For this review, take the finished solid that the model builds, in its own axes (mm). Round coordinates to 2 decimals unless told otherwise and drop trailing zeros. Write each loop counter-clockwise with the first axis right and the second up, starting at its lowest first coordinate (ties: lowest second). Pieces come first, ordered by that corner, then holes. Notation, with made-up numbers: M -11.75,-19.5 L 18.25,-19.5 A6 ccw 18.25,-15.5 Z; hole C -27.75,24 d7. An arc over 180 degrees is marked long. One line per question, with ' | ' between items.
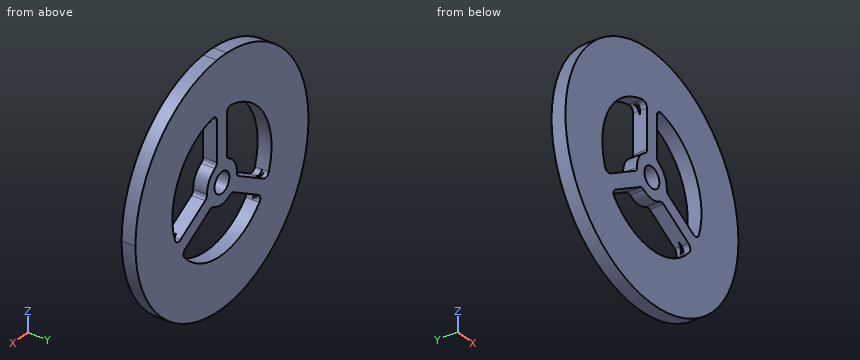
```python
from build123d import *

# Parameters (mm, degrees)
F0_R     = 1.5
F1_DEPTH = 1


with BuildPart() as f1:
    # F0 (on Front) → F1 (new body, symmetric)
    with BuildSketch(Plane.XZ):
        with BuildLine():
            ThreePointArc((-1, 17.412308), (-11.973877, -12.681275), (17.441, 0))
            ThreePointArc((17.441, 0), (12.681275, 11.973877), (1, 17.412308))
            ThreePointArc((1, 17.412308), (0, 17.441), (-1, 17.412308))
        make_face()
        with BuildLine():
            ThreePointArc((-2.373679, -2.525145), (-1.983172, -2.424438), (-1.596733, -2.539773))
            ThreePointArc((-1.596733, -2.539773), (0, -3), (1.596733, -2.539773))
            ThreePointArc((1.596733, -2.539773), (1.983172, -2.424438), (2.373679, -2.525145))
            Line((2.373679, -2.525145), (7.363259, -5.40588))
            ThreePointArc((7.363259, -5.40588), (7.729194, -5.933007), (7.555614, -6.550779))
            ThreePointArc((7.555614, -6.550779), (0, -10), (-7.555614, -6.550779))
            ThreePointArc((-7.555614, -6.550779), (-7.729194, -5.933007), (-7.363259, -5.40588))
            Line((-7.363259, -5.40588), (-2.373679, -2.525145))
        make_face(mode=Mode.SUBTRACT)
        with BuildLine():
            ThreePointArc((-9.450948, -3.267964), (-8.660254, 5), (-1.895334, 9.818743))
            ThreePointArc((-1.895334, 9.818743), (-1.273538, 9.660182), (-1, 9.079709))
            Line((-1, 9.079709), (-1, 3.318238))
            ThreePointArc((-1, 3.318238), (-1.108039, 2.929697), (-1.401141, 2.652697))
            ThreePointArc((-1.401141, 2.652697), (-2.598076, 1.5), (-2.997874, -0.112925))
            ThreePointArc((-2.997874, -0.112925), (-3.091211, -0.505258), (-3.373679, -0.793094))
            Line((-3.373679, -0.793094), (-8.363259, -3.673829))
            ThreePointArc((-8.363259, -3.673829), (-9.002732, -3.727174), (-9.450948, -3.267964))
        make_face(mode=Mode.SUBTRACT)
        Circle(F0_R, mode=Mode.SUBTRACT)
        with BuildLine():
            Line((1, 3.318238), (1, 9.079709))
            ThreePointArc((1, 9.079709), (1.273538, 9.660182), (1.895334, 9.818743))
            ThreePointArc((1.895334, 9.818743), (8.660254, 5), (9.450948, -3.267964))
            ThreePointArc((9.450948, -3.267964), (9.002732, -3.727174), (8.363259, -3.673829))
            Line((8.363259, -3.673829), (3.373679, -0.793094))
            ThreePointArc((3.373679, -0.793094), (3.091211, -0.505258), (2.997874, -0.112925))
            ThreePointArc((2.997874, -0.112925), (2.598076, 1.5), (1.401141, 2.652697))
            ThreePointArc((1.401141, 2.652697), (1.108039, 2.929697), (1, 3.318238))
        make_face(mode=Mode.SUBTRACT)
    extrude(amount=F1_DEPTH, both=True)

    # F2 (on Right) → F3 (revolve, cut)
    with BuildSketch(Plane.YZ):
        Polygon((0.4216, 9.94), (0, 10), (0, 8.5), align=None)
    revolve(axis=Axis((0, -2.204443, 0), (0, 1, 0)), mode=Mode.SUBTRACT)


solid = f1.part
```
Item 1: To check wall thickness, follow line 1 along X through (y, z) = (0.6, -3.5); line 2 along Z through (x, y) = (-0.5, -0.25); line 3 along X through (y, z) = (0.25, 3). State the ranges of each line that lie inside material, in increasing order. Write a range as from..to.
Results:
line 1: -17.09..-9.32, -8.06..-4.06, 4.06..8.06, 9.32..17.09 | line 2: -17.43..-9.99, -2.96..-1.41, 1.41..17.43 | line 3: -17.18..-9.54, -1.07..1.07, 9.54..17.18
Item 2: Take a section at B-B (z = -14). Write out the cut boundary in (x, y), then the cut area to 3 significant figures.
Results:
outline: M -10.4,-1 L 10.4,-1 L 10.4,1 L -10.4,1 Z | area: 41.6 mm2
Item 3: Insertion check: pin 1 Ø1 at (y, z) = (0.5, 7.5) entering from -X; pin 2 Ø1 at (x, y) = (10.5, 0) entering from -Z; pin 3 Ø2.5 at (x, z) = (0, 0) entering from +Y; pin 4 Ø1 at (y, z) = (-0.5, -9.5) entering from +X. Each pin has a flat end and moves straight along its axis. Give the tip position at first contact, or say it passes through.
Results:
pin 1: x = -15.97 | pin 2: z = -14.29 | pin 3: through | pin 4: x = 14.94
Item 4: Take a section at C-C (x = 11). Write out the cut boundary in (y, z), then the cut area to 3 significant figures.
Results:
outline: M -1,-13.53 L 1,-13.53 L 1,13.53 L -1,13.53 Z | area: 54.1 mm2
Item 5: Take a section at A-A (y = -0.65). Write out the cut boundary in (x, z).
Results:
outline: M -1,17.41 A17.44 ccw long 1,17.41 A17.44 ccw Z; hole M -9.45,-3.27 A0.75 ccw -8.36,-3.67 L -3.37,-0.79 A0.75 ccw -3,-0.11 A3 cw -1.4,2.65 A0.75 ccw -1,3.32 L -1,9.08 A0.75 ccw -1.9,9.82 A10 ccw Z; hole M -7.56,-6.55 A10 ccw 7.56,-6.55 A0.75 ccw 7.36,-5.41 L 2.37,-2.53 A0.75 ccw 1.6,-2.54 A3 cw -1.6,-2.54 A0.75 ccw -2.37,-2.53 L -7.36,-5.41 A0.75 ccw Z; hole C 0,0 d3; hole M 1,3.32 A0.75 ccw 1.4,2.65 A3 cw 3,-0.11 A0.75 ccw 3.37,-0.79 L 8.36,-3.67 A0.75 ccw 9.45,-3.27 A10 ccw 1.9,9.82 A0.75 ccw 1,9.08 Z
